For this review, take the finished solid that the model builds, in its own axes (mm). Face numbers are marked on the shaded views. A direction names the side the tool comes from. Coordinates: 2 decimals unless noted, no trailing zeros. Loops run counter-clockwise (first coordinate to the right, second up) from the corner with the lowest first, then second, coordinate; pieces in that order, holes last. Notation, with made-up numbers: M -25,80 L -6,80 A25 ccw -6,116 Z; hole C -26.75,71 d3. An arc over 180 degrees is marked long. Put each result on its own line as item: value.
```python
from build123d import *

# Parameters (mm, degrees)
F0_R         = 8
F1_DEPTH     = 10
F2_R         = 1.5
F3_DEPTH     = 22.1
F4_R         = 1.4
F5_DEPTH     = 8
F6_T1_DEPTH  = 25.4217528018
F7_R         = 2
F8_R         = 2
F10_DEPTH    = 2.5
F11_R        = 4
F12_DEPTH    = 6
F14_DEPTH    = 2.5
F15_T1_DEPTH = 9.0773234724
F17_DEPTH    = 25
F18_DEPTH    = 7.25


# Not quite as in the source:
# - a fillet or chamfer that OpenCascade refuses, or shapes differently, is made with other operations: its cross-section is extruded or revolved along the edge and cut away or added


with BuildPart() as f1:
    # F0 (on Front) → F1 (new body)
    with BuildSketch(Plane.XZ):
        with BuildLine():
            ThreePointArc((-5.123475383, -8), (4.5594398703, -8.3343570879), (9.5, 0))
            ThreePointArc((9.5, 0), (2.5991730895, 9.1375215048), (-8.0777472107, 5))
            ThreePointArc((-8.0777472107, 5), (-8.4879541617, 4.2666888975), (-8.8317608663, 3.5))
            ThreePointArc((-8.8317608663, 3.5), (-9.0415515645, -2.9155351664), (-5.123475383, -8))
        make_face()
        Circle(F0_R, mode=Mode.SUBTRACT)
        with BuildLine():
            ThreePointArc((-8.8317608663, 3.5), (-8.4879541617, 4.2666888975), (-8.0777472107, 5))
            Line((-8.0777472107, 5), (-23.5, 5))
            ThreePointArc((-23.5, 5), (-24.7247448714, 4.5811388301), (-25.4364916731, 3.5))
            Line((-25.4364916731, 3.5), (-8.8317608663, 3.5))
        make_face()
        with BuildLine():
            Line((-23.5, -8), (-5.123475383, -8))
            ThreePointArc((-5.123475383, -8), (-9.0415515645, -2.9155351664), (-8.8317608663, 3.5))
            Line((-8.8317608663, 3.5), (-25.4364916731, 3.5))
            ThreePointArc((-25.4364916731, 3.5), (-25.4840593925, 3.252008585), (-25.5, 3))
            Line((-25.5, 3), (-25.5, 0))
            Line((-25.5, 0), (-25.5, -3.5))
            Line((-25.5, -3.5), (-25.5, -6))
            ThreePointArc((-25.5, -6), (-24.9142135624, -7.4142135624), (-23.5, -8))
        make_face()
        with BuildLine():
            ThreePointArc((-25.5, 3), (-25.4840593925, 3.252008585), (-25.4364916731, 3.5))
            Line((-25.4364916731, 3.5), (-25.5, 3.5))
            Line((-25.5, 3.5), (-31.5, 3.5))
            ThreePointArc((-31.5, 3.5), (-32.2071067812, 3.2071067812), (-32.5, 2.5))
            Line((-32.5, 2.5), (-32.5, 1.5))
            Line((-32.5, 1.5), (-32.5, 0))
            Line((-32.5, 0), (-32.5, -1.5))
            Line((-32.5, -1.5), (-32.5, -2.5))
            ThreePointArc((-32.5, -2.5), (-32.2071067812, -3.2071067812), (-31.5, -3.5))
            Line((-31.5, -3.5), (-25.5, -3.5))
            Line((-25.5, -3.5), (-25.5, 0))
            Line((-25.5, 0), (-25.5, 3))
        make_face()
    extrude(amount=F1_DEPTH)

    # F2 (on face) → F3 (cut)
    with BuildSketch(Plane(origin=(-32.5, 0, 0), x_dir=(0, -1, 0), z_dir=(-1, 0, 0))):
        with Locations((5, 0)):
            Circle(F2_R)
    extrude(amount=-F3_DEPTH, mode=Mode.SUBTRACT)

    # F4 (on face) → F5 (cut)
    with BuildSketch(Plane(origin=(0, 0, -8), x_dir=(1, 0, 0), z_dir=(0, 0, -1))):
        with Locations((-12.4, 5)):
            Circle(F4_R)
        with Locations((-19.5, 5)):
            Circle(F4_R)
    extrude(amount=-F5_DEPTH, mode=Mode.SUBTRACT)

    # F6: fillet of radius 2 on 2 edges, made by hand

    # F6_s2 → F6_t1 (cut)
    with BuildSketch(Plane.YZ.offset(-28.4997500063)):
        with BuildLine():
            ThreePointArc((-8.0001, 5.0001), (-9.4143135624, 4.4143135624), (-10.0001, 3.0001))
            Line((-10.0001, 3.0001), (-10.0401, 3.0001))
            ThreePointArc((-10.0401, 3.0001), (-10.04, 4.00005), (-10.04, 5))
            Line((-10.04, 5), (-10, 5.04))
            ThreePointArc((-10, 5.04), (-9.00005, 5.04), (-8.0001, 5.0401))
            Line((-8.0001, 5.0401), (-8.0001, 5.0001))
        make_face()
        with BuildLine():
            ThreePointArc((-1.9999, 5.0001), (-0.5856864376, 4.4143135624), (0.0001, 3.0001))
            Line((0.0001, 3.0001), (0.0401, 3.0001))
            ThreePointArc((0.0401, 3.0001), (0.04, 4.00005), (0.04, 5))
            Line((0.04, 5), (0, 5.04))
            ThreePointArc((0, 5.04), (-0.99995, 5.04), (-1.9999, 5.0401))
            Line((-1.9999, 5.0401), (-1.9999, 5.0001))
        make_face()
    extrude(amount=F6_T1_DEPTH, mode=Mode.SUBTRACT)

    # F7
    f7_edges = [f1.edges().sort_by_distance(p)[0] for p in [
        (-32.5, -10, 0),
        (-32.5, 0, 0),
    ]]
    fillet(f7_edges, radius=F7_R)

    # F8
    f8_edges = [f1.edges().sort_by_distance(p)[0] for p in [
        (-14.311738, -10, -8),
        (-14.311738, 0, -8),
    ]]
    fillet(f8_edges, radius=F8_R)

    # F9 (on Front) → F10 (join)
    with BuildSketch(Plane.XZ):
        with BuildLine():
            ThreePointArc((0.8300844627, 8.6718317984), (6.4467419184, 5.8591147448), (8.7114698505, 0))
            Line((8.7114698505, 0), (14.25, 0))
            ThreePointArc((14.25, 0), (16.5494157481, 5.0749187005), (21.8810517975, 6.6922528143))
            Line((21.8810517975, 6.6922528143), (1.6475767802, 9.3560403352))
            Line((1.6475767802, 9.3560403352), (0.8300844627, 9.4636652405))
            Line((0.8300844627, 9.4636652405), (0.8300844627, 8.6718317984))
        make_face()
        with BuildLine():
            Line((14.25, 0), (8.7114698505, 0))
            ThreePointArc((8.7114698505, 0), (6.4467419184, -5.8591147448), (0.8300844627, -8.6718317984))
            Line((0.8300844627, -8.6718317984), (0.8300844627, -9.4636652405))
            Line((0.8300844627, -9.4636652405), (1.6475767802, -9.3560403352))
            Line((1.6475767802, -9.3560403352), (21.8810517975, -6.6922528143))
            ThreePointArc((21.8810517975, -6.6922528143), (16.5494157481, -5.0749187005), (14.25, 0))
        make_face()
        with BuildLine():
            ThreePointArc((21.8810517975, 6.6922528143), (16.5494157481, 5.0749187005), (14.25, 0))
            Line((14.25, 0), (21, 0))
            Line((21, 0), (21.8810517975, -6.6922528143))
            ThreePointArc((21.8810517975, -6.6922528143), (26.0749187005, -4.4505842519), (27.75, 0))
            ThreePointArc((27.75, 0), (26.0749187005, 4.4505842519), (21.8810517975, 6.6922528143))
        make_face()
        with BuildLine():
            Line((21, 0), (14.25, 0))
            ThreePointArc((14.25, 0), (16.5494157481, -5.0749187005), (21.8810517975, -6.6922528143))
            Line((21.8810517975, -6.6922528143), (21, 0))
        make_face()
        with BuildLine():
            Line((1.6475767802, -9.3560403352), (0.8300844627, -9.4636652405))
            ThreePointArc((0.8300844627, -9.4636652405), (1.2399988261, -9.4187261831), (1.6475767802, -9.3560403352))
        make_face()
        with BuildLine():
            ThreePointArc((1.6475767802, 9.3560403352), (1.2399988261, 9.4187261831), (0.8300844627, 9.4636652405))
            Line((0.8300844627, 9.4636652405), (1.6475767802, 9.3560403352))
        make_face()
    extrude(amount=F10_DEPTH)

    # F11 (on face) → F12 (join)
    with BuildSketch(Plane.XZ.offset(2.5)):
        with Locations((21, 0)):
            Circle(F11_R)
    extrude(amount=F12_DEPTH)

    # F13 (on face) → F14 (join)
    with BuildSketch(Plane.XZ.offset(2.5)):
        with BuildLine():
            Line((14.25, -7.6968998426), (14.25, 0))
            Line((14.25, 0), (14.25, 7.6968998426))
            Line((14.25, 7.6968998426), (1.6475767802, 9.3560403352))
            Line((1.6475767802, 9.3560403352), (1.6475767802, 8.3387943225))
            ThreePointArc((1.6475767802, 8.3387943225), (8.5, 0), (1.6475767802, -8.3387943225))
            Line((1.6475767802, -8.3387943225), (1.6475767802, -9.3560403352))
            Line((1.6475767802, -9.3560403352), (14.25, -7.6968998426))
        make_face()
    extrude(amount=F14_DEPTH)

    # F15: fillet of radius 3 on 2 edges, made by hand

    # F15_s2 → F15_t1 (cut)
    with BuildSketch(Plane.XZ.offset(2.5)):
        with BuildLine():
            ThreePointArc((11.6415785767, 8.0403050378), (13.5055194224, 7.044007899), (14.25, 5.0659704537))
            Line((14.25, 5.0659704537), (14.25, 7.6968998426))
            Line((14.25, 7.6968998426), (11.6415785767, 8.0403050378))
        make_face()
        with BuildLine():
            ThreePointArc((14.25, -5.0659704537), (13.5055194224, -7.044007899), (11.6415785767, -8.0403050378))
            Line((11.6415785767, -8.0403050378), (14.25, -7.6968998426))
            Line((14.25, -7.6968998426), (14.25, -5.0659704537))
        make_face()
    extrude(amount=F15_T1_DEPTH, mode=Mode.SUBTRACT)

    # F16 (on face) → F17 (cut)
    with BuildSketch(Plane.XZ.offset(10)):
        with BuildLine():
            Line((-37.4530367553, -9.75), (0, -9.75))
            ThreePointArc((0, -9.75), (9.75, 0), (0, 9.75))
            Line((0, 9.75), (0, 13.4185552597))
            Line((0, 13.4185552597), (-34.6982963383, 13.4185552597))
            Line((-34.6982963383, 13.4185552597), (-37.4530367553, 13.4185552597))
            Line((-37.4530367553, 13.4185552597), (-37.4530367553, -9.75))
        make_face()
    extrude(amount=-F17_DEPTH, mode=Mode.SUBTRACT)

    # F18 (cut): a face of the model
    f18_faces = [f1.faces().sort_by_distance(p)[0] for p in [
        (21, -8.5, 0),
    ]]
    extrude(f18_faces, amount=-F18_DEPTH, mode=Mode.SUBTRACT)


solid = f1.part
```
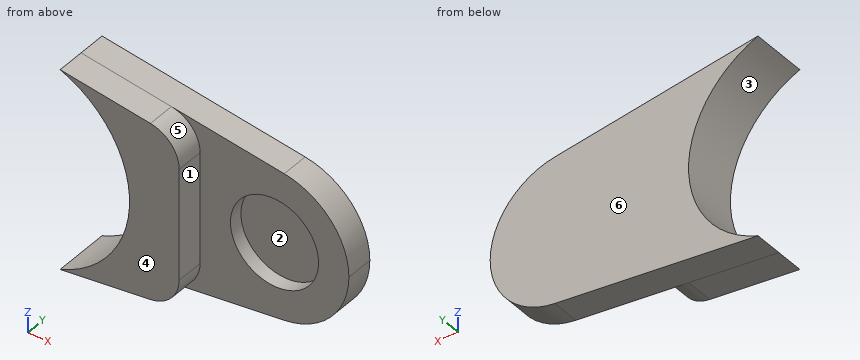
(1) Wall thickness on line 1 along Y through (x, z) = (21.75, 5.25); line 2 along Z through (x, y) = (6, -0.7); line 3 along Z through (x, y) = (21, -2.1): over which ranges is each line inside the solid? List them lowest first. Write a range as [from, to].
Determined:
line 1: y = [-2.5, 0]
line 2: z = [-8.78, -7.69], [7.69, 8.78]
line 3: z = [-6.81, -4], [4, 6.81]
(2) For pin 1 (1.5 mm diameter, centred on y = -3, z = 3, fed in from +X); pin 2 (1.5 mm diameter, centred on x = 20, y = -2, fed in from +Z); pin 3 (5 mm diameter, centred on x = 8, z = 2.5, fed in from +Y); pin 4 (1 mm diameter, centred on x = 18, y = -4.5, fed in from -Z), all flat-tipped, find the tip position at first contact; note any pin that passes through.
Determined:
pin 1: stops at x = 27.29
pin 2: stops at z = 7.04
pin 3: stops at y = 0
pin 4: passes through
(3) Add section B-B (x = 6.5). Write out the cut boundary in (y, z), plus the area to 3 significant figures.
Determined:
outline: M -5,-8.72 L 0,-8.72 L 0,-7.27 L -5,-7.27 Z; M -5,7.27 L 0,7.27 L 0,8.72 L -5,8.72 Z
area: 14.5 mm^2
(4) Add section C-C (z = -2). Write out the cut boundary in (x, y), plus the area to 3 significant figures.
Determined:
outline: M 9.54,-5 L 14.25,-5 L 14.25,-2.5 L 17.54,-2.5 L 17.54,-1.25 L 24.46,-1.25 L 24.46,-2.5 L 27.45,-2.5 L 27.45,0 L 9.54,0 Z
area: 47.9 mm^2
(5) Add section D-D (y = -4.4). Write out the cut boundary in (x, z), plus the area to 3 significant figures.
Determined:
outline: M 3.45,-9.12 L 11.64,-8.04 A3 ccw 14.25,-5.07 L 14.25,5.07 A3 ccw 11.64,8.04 L 3.45,9.12 A9.75 cw Z
area: 95.3 mm^2
(6) Add section A-A (y = -1.9). Write out the cut boundary in (x, z).
Determined:
outline: M 3.45,-9.12 L 21.88,-6.69 A6.75 ccw 21.88,6.69 L 3.45,9.12 A9.75 cw Z; hole C 21,0 d8
(7) Tool access review of the marked faces 5 and 6: name each direction out of +Z, -Z, +X, -X, +Y, -Y from which nothing blocks a thin tool from reaching the whole face with its end or side.
Determined:
face 5: +Z, +X, -Y
face 6: +Z, -Z, +X, -X, +Y
(8) Draft analysis for pull direction X (two halves, no side actions). For the marked faces 1, 2, 3 and 4, state which applies: +X half, -X half, draft (parallel to the pull), parting line (faces both ways), or undercut.
Determined:
face 1: +X half
face 2: undercut
face 3: -X half
face 4: draft
